```python
from build123d import *

# Parameters (mm, degrees)
SKETCH_1_R          = 57.5
EXTRUDE_1_DEPTH     = 26
FILLET_2_R          = 7
CUT_EXTRUDE_1_DEPTH = 8.5
SKETCH_3_R          = 1.5
CUT_EXTRUDE_3_DEPTH = 91.5
SKETCH_3_4_R        = 3
CUT_EXTRUDE_4_DEPTH = 14
CUT_EXTRUDE_START   = 15
SKETCH_3_6_R        = 3
CUT_EXTRUDE_5_DEPTH = 67
FILLET_10_R         = 3
FILLET_11_R         = 3
FILLET_12_R         = 3
FILLET_13_R         = 3
CUT_EXTRUDE_START_2 = 16
SKETCH_3_8_R        = 3
CUT_EXTRUDE_6_DEPTH = 10
EXTRUDE_START       = 26
SKETCH_3_21_R       = 11.5
EXTRUDE_3_DEPTH     = 7
FILLET_30_R         = 7
SKETCH_3_22_R       = 11.5
EXTRUDE_4_DEPTH     = 7
SKETCH_3_23_R       = 11.5
EXTRUDE_5_DEPTH     = 7
FILLET_32_R         = 7
FILLET_33_R         = 7


with BuildPart() as part:
    # Эскиз1 → Бобышка-Вытянуть1 (new body)
    with BuildSketch(Plane.XY):
        with Locations(Location((0, 0, 0), (0, 0, 180))):
            Circle(SKETCH_1_R)
    extrude(amount=EXTRUDE_1_DEPTH)

    # Скругление2
    fillet_2_edges = [part.edges().sort_by_distance(p)[0] for p in [
        (57.5, 0, 0),
        (57.5, 0, 26),
    ]]
    fillet(fillet_2_edges, radius=FILLET_2_R)

    # Эскиз2 → Вырез-Вытянуть1 (cut)
    with BuildSketch(Plane.XY):
        Polygon((0, 26), (-8, 26), (-8, 43), (8, 43), (8, 26), align=None)
    extrude(amount=CUT_EXTRUDE_1_DEPTH, mode=Mode.SUBTRACT)

    # Эскиз3 → Вырез-Вытянуть3 (cut)
    with BuildSketch(Plane.XY):
        with Locations((0, 35)):
            Circle(SKETCH_3_R)
    extrude(amount=CUT_EXTRUDE_3_DEPTH, mode=Mode.SUBTRACT)

    # Эскиз3<4> → Вырез-Вытянуть4 (cut)
    with BuildSketch(Plane.XY):
        with Locations((0, 35)):
            Circle(SKETCH_3_4_R)
    extrude(amount=CUT_EXTRUDE_4_DEPTH, mode=Mode.SUBTRACT)

    # Эскиз3<6> → Вырез-Вытянуть5 (cut)
    with BuildSketch(Plane.XY.offset(CUT_EXTRUDE_START)):
        with Locations((0, 35)):
            Circle(SKETCH_3_6_R)
    extrude(amount=CUT_EXTRUDE_5_DEPTH, mode=Mode.SUBTRACT)

    # Скругление10
    fillet_10_edges = [part.edges().sort_by_distance(p)[0] for p in [
        (8, 43, 4.25),
    ]]
    fillet(fillet_10_edges, radius=FILLET_10_R)

    # Скругление11
    fillet_11_edges = [part.edges().sort_by_distance(p)[0] for p in [
        (-8, 43, 4.25),
    ]]
    fillet(fillet_11_edges, radius=FILLET_11_R)

    # Скругление12
    fillet_12_edges = [part.edges().sort_by_distance(p)[0] for p in [
        (-8, 26, 4.25),
    ]]
    fillet(fillet_12_edges, radius=FILLET_12_R)

    # Скругление13
    fillet_13_edges = [part.edges().sort_by_distance(p)[0] for p in [
        (8, 26, 4.25),
    ]]
    fillet(fillet_13_edges, radius=FILLET_13_R)

    # Эскиз3<8> → Вырез-Вытянуть6 (cut)
    with BuildSketch(Plane.XY.offset(CUT_EXTRUDE_START_2)):
        with Locations((0, 35)):
            Circle(SKETCH_3_8_R)
        with Locations((30.310889132, -17.5)):
            Circle(SKETCH_3_8_R)
        with Locations((-30.310889132, -17.5)):
            Circle(SKETCH_3_8_R)
    extrude(amount=CUT_EXTRUDE_6_DEPTH, mode=Mode.SUBTRACT)

    # Эскиз3<21> → Бобышка-Вытянуть3 (add)
    with BuildSketch(Plane.XY.offset(EXTRUDE_START)):
        with Locations((-22.516660498, 13)):
            Circle(SKETCH_3_21_R)
    extrude(amount=EXTRUDE_3_DEPTH)

    # Скругление30
    fillet_30_edges = [part.edges().sort_by_distance(p)[0] for p in [
        (-34.016660498, 13, 33),
    ]]
    fillet(fillet_30_edges, radius=FILLET_30_R - 0.0001)  # a hair under: the kernel refuses the full size

    # Эскиз3<22> → Бобышка-Вытянуть4 (add)
    with BuildSketch(Plane.XY.offset(EXTRUDE_START)):
        with Locations((22.516660498, 13)):
            Circle(SKETCH_3_22_R)
    extrude(amount=EXTRUDE_4_DEPTH)

    # Эскиз3<23> → Бобышка-Вытянуть5 (add)
    with BuildSketch(Plane.XY.offset(EXTRUDE_START)):
        with Locations((0, -26)):
            Circle(SKETCH_3_23_R)
    extrude(amount=EXTRUDE_5_DEPTH)

    # Скругление32
    fillet_32_edges = [part.edges().sort_by_distance(p)[0] for p in [
        (11.016660498, 13, 33),
    ]]
    fillet(fillet_32_edges, radius=FILLET_32_R - 0.0001)  # a hair under: the kernel refuses the full size

    # Скругление33
    fillet_33_edges = [part.edges().sort_by_distance(p)[0] for p in [
        (-11.5, -26, 33),
    ]]
    fillet(fillet_33_edges, radius=FILLET_33_R - 0.0001)  # a hair under: the kernel refuses the full size


solid = part.part
```
For this review, take the finished solid that the model builds, in its own axes (mm). A direction names the side the tool comes from. Coordinates: 2 decimals unless noted, no trailing zeros. Order: outer loops, then holes, each group sorted by start corner. A loop starts at its lowest first (then second) coordinate and runs counter-clockwise, first axis right, second up. Notation, with made-up numbers: (3.5, 30.25) -> (12.5, 30.25) arc R28 ccw to (12.5, 52.25) -> close; hole circle Ø1 at (-19.5, -31.75). An arc over 180 degrees is marked (long way). Use CSV: the item, a comma, the result in double quotes. Start each with the question number.
Item 1: We need section A-A, the plane y = 0. Give the boundary of the cut face in (x, z), then the cut area to 3 significant figures.
Item 2: We need section B-B, the plane z = 2.5. Give the boundary of the cut face in (x, y).
Item 3: We need section D-D, the plane z = 10.5. Give the boundary of the cut face in (x, y), then the cut area to 3 significant figures.
Item 4: For faces 3 (the face through (27.93, -19.325, 20.93)), 4 (the face through (0, -26, 33)), 5 (the face through (0, 43, 4)), list the 3-axis set-ups (+Z, -Z, +X, -X, +Y, -Y) from which the entire face can be reached by the end or side of a thin tool; tool diameter is ignored.
Item 5: Draft analysis for pull direction Y (two halves, no side actions). For faces 1 (the face through (-23, 13, 33)), 2 (the face through (7.14, 42.1, 4.31)), state which applies: pulls with the +Y half, pulls with the -Y half, needs draft (parallel to the pull), parting line crosses it, or undercut.
Item 6: We need section C-C, the plane z = 24.5. Give the boundary of the cut face in (x, y), then the cut area to 3 significant figures.
Item 7: Wall thickness on probe 1 along Y at (x, z) = (0, 11); probe 2 along Z at (x, y) = (-14.5, -9); probe 3 along X at (y, z) = (35, 14.7): over which ranges is each line inside the solid? List them lowest first.
Item 8: Insertion check: pin 1 (7 mm diameter, centred on x = -1, z = 3, fed in from -Y); pin 2 (4 mm diameter, centred on y = 33.5, z = 2.5, fed in from -X); pin 3 (1 mm diameter, centred on y = -22.5, z = 19.5, fed in from +X). Each pin has a flat end and moves straight along its axis. Give the tip position at first contact, or say it passes through.
Derived:
1,outline,"(-57.5, 7) arc R7 ccw to (-50.5, 0) -> (50.5, 0) arc R7 ccw to (57.5, 7) -> (57.5, 19) arc R7 ccw to (50.5, 26) -> (-50.5, 26) arc R7 ccw to (-57.5, 19) -> close"
1,area,"2,950 mm^2"
2,outline,"circle Ø111.72 at (0, 0); hole (-8, 29) arc R3 ccw to (-5, 26) -> (5, 26) arc R3 ccw to (8, 29) -> (8, 40) arc R3 ccw to (5, 43) -> (-5, 43) arc R3 ccw to (-8, 40) -> close"
3,outline,"circle Ø115 at (0, 0); hole circle Ø6 at (0, 35)"
3,area,"10,400 mm^2"
4,face 3,"+Z"
4,face 4,"+Z, +X, -X, +Y, -Y"
4,face 5,"-Z"
5,face 1,"needs draft"
5,face 2,"undercut"
6,outline,"circle Ø109.66 at (0, 0); hole circle Ø6 at (-30.31, -17.5); hole circle Ø6 at (0, 35); hole circle Ø6 at (30.31, -17.5)"
6,area,"9,360 mm^2"
7,probe 1,"y = -57.5 to 32, 38 to 57.5"
7,probe 2,"z = 0 to 26"
7,probe 3,"x = -45.62 to -1.5, 1.5 to 45.62"
8,pin 1,"stops at y = -57.48"
8,pin 2,"stops at x = -46.85"
8,pin 3,"stops at x = 53.11"
